Geometry: see drawing. Coordinates: mm, zero at the bounding-box minimum. A direction names the side the tool comes from. Round coordinates to 2 decimals unless told otherwise and drop trailing zeros. Loops run counter-clockwise (first coordinate to the right, second up) from the corner with the lowest first, then second, coordinate; pieces in that order, holes last. Notation, with made-up numbers: (72.25, 63.5) - (100.25, 63.5) arc R25 cw to (100.25, 96.5) - close; hole circle Ø9 at (85.25, -19.5). An arc over 180 degrees is marked (long way). Answer in a Markdown table with one row per item. Add a question column.
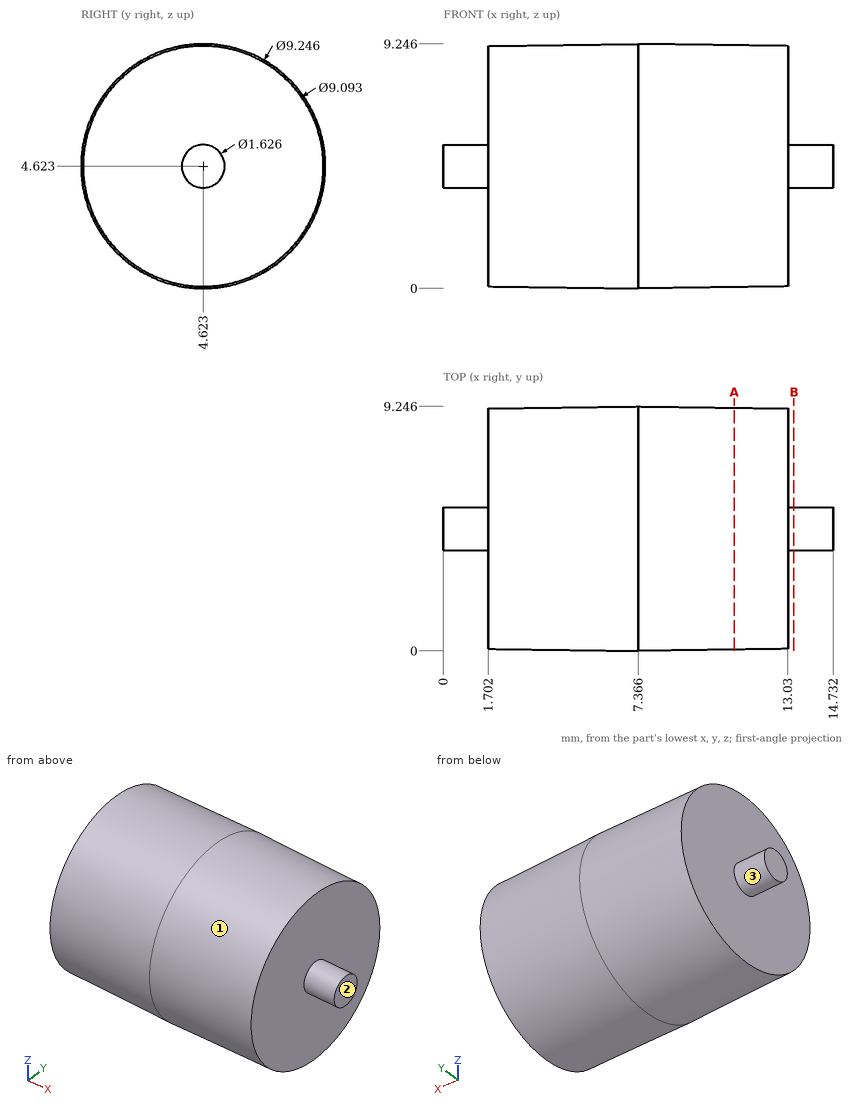
1) Section B-B, the plane x = 13.25. Return the cut outline in (y, z) (1 decimal).
2) Section A-A, the plane x = 11. Return the cut outline in (y, z).
3) Reachability of the marked faces 1, 2 and 3 from +Z, -Z, +X, -X, +Y, -Y: full face, straight path, thin tool, end or side. Return the list, or none.
4) Contact query for flat-ended pins moving along their axis: pin 1 Ø1 at (x, z) = (4.5, 2) entering from -Y; pin 2 Ø1 at (y, z) = (3.5, 6.5) entering from -X; pin 3 Ø2 at (x, y) = (4, 5.5) entering from +Z. Output: stop coordinate, or through.
5) Material intervals for line 1 along X through (y, z) = (5, 2.5); line 2 along Y through (x, z) = (2.75, 5); line 3 along Y through (x, z) = (4.5, 2.5) (1 decimal), sorted ascending. Write a range as from..to.
Evaluation:
| question | item | result |
|---|---|---|
| 1 | outline | circle Ø1.6 at (4.6, 4.6) |
| 2 | outline | circle Ø9.15 at (4.62, 4.62) |
| 3 | face 1 | +X |
| 3 | face 2 | +Z, -Z, +X, +Y, -Y |
| 3 | face 3 | -X |
| 4 | pin 1 | stops at y = 0.56 |
| 4 | pin 2 | stops at x = 1.7 |
| 4 | pin 3 | stops at z = 9.21 |
| 5 | line 1 | x = 1.7..13.03 |
| 5 | line 2 | y = 0.08..9.17 |
| 5 | line 3 | y = 0.6..8.7 |
